CAD build for the part. Positions are in the model's coordinates, mm. Coordinates: 2 decimals unless noted, no trailing zeros. Write each loop counter-clockwise with the first axis right and the second up, starting at its lowest first coordinate (ties: lowest second). Pieces come first, ordered by that corner, then holes. Notation, with made-up numbers: (59.5, 61) -> (107.5, 61) arc R22 cw to (107.5, 92) -> close; hole circle Ø3 at (-24.5, 74.5). An arc over 180 degrees is marked (long way). Answer as CSV lines item,"result".
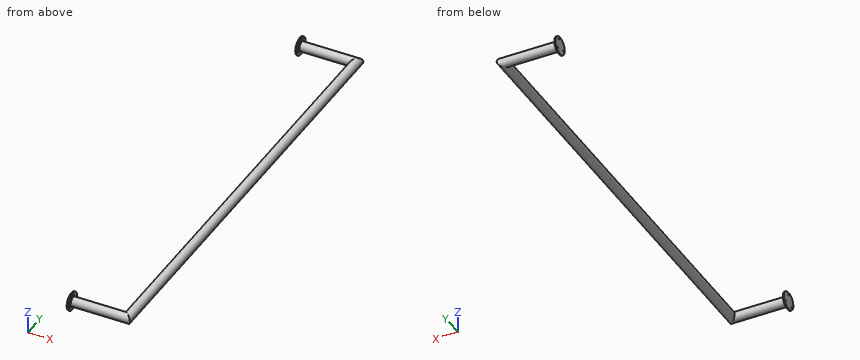
```python
from build123d import *

# Parameters (mm, degrees)
F0_R     = 21
F0_R_2   = 20
F3_R     = 40
F3_R_2   = 3.25
F4_DEPTH = 5
F5_SIZE  = 2
F6_SIZE  = 3


with BuildPart() as f2:
    # F2: sweep along a path in F1
    with BuildLine(Plane.XY) as f2_path:
        Line((0, 0), (250, 0))
        Line((250, 0), (250, -1948.319))
        Line((250, -1948.319), (0, -1948.319))
    # F0 (on Right) → F2 (sweep)
    with BuildSketch(Plane.YZ):
        Circle(F0_R)
        Circle(F0_R_2, mode=Mode.SUBTRACT)
    sweep(path=f2_path.line, transition=Transition.RIGHT)

    # F3 (on face) → F4 (join)
    with BuildSketch(Plane(origin=(0, 0, 0), x_dir=(0, -1, 0), z_dir=(-1, 0, 0))):
        with Locations((1948.319, 0)):
            Circle(F3_R)
        with Locations((1921.9052251846, -15.25)):
            Circle(F3_R_2, mode=Mode.SUBTRACT)
        with Locations((1974.7327748154, -15.25)):
            Circle(F3_R_2, mode=Mode.SUBTRACT)
        with Locations((1948.319, 30.5)):
            Circle(F3_R_2, mode=Mode.SUBTRACT)
        Circle(F3_R)
        with Locations((-21.187080299, -21.9398639103)):
            Circle(F3_R_2, mode=Mode.SUBTRACT)
        with Locations((29.5940196514, -7.3786178158)):
            Circle(F3_R_2, mode=Mode.SUBTRACT)
        with Locations((-8.4069393524, 29.3184817261)):
            Circle(F3_R_2, mode=Mode.SUBTRACT)
    extrude(amount=-F4_DEPTH)

    # F5
    f5_edges = [f2.edges().sort_by_distance(p)[0] for p in [
        (5, 11.656939, 29.318482),
        (5, -26.34402, -7.378618),
        (5, 24.43708, -21.939864),
        (5, -1945.069, 30.5),
        (5, -1971.482775, -15.25),
        (5, -1918.655225, -15.25),
    ]]
    chamfer(f5_edges, length=F5_SIZE)

    # F6
    f6_edges = [f2.edges().sort_by_distance(p)[0] for p in [
        (5, -21, 0),
        (5, -1927.319, 0),
    ]]
    chamfer(f6_edges, length=F6_SIZE)


solid = f2.part
```
Item 1: Saw through at B-B on y = -1611. Give the cut face in (x, z), and give its area (3 significant figures).
Answer below:
outline,"circle Ø42 at (250, 0); hole circle Ø40 at (250, 0)"
area,"129 mm2"
Item 2: Saw through at A-A on x = 158. Give the cut face in (y, z).
Answer below:
outline,"circle Ø42 at (-1948.32, 0); circle Ø42 at (0, 0); hole circle Ø40 at (-1948.32, 0); hole circle Ø40 at (0, 0)"
Item 3: Flat gauge pins, fed straight in: pin 1 (8 mm diameter, centred on y = -572.5, z = -19, fed in from -X); pin 2 (6 mm diameter, centred on y = -1428.5, z = 3, fed in from -X); pin 3 (1.5 mm diameter, centred on y = -1363, z = -3, fed in from -X). Where does each tip first touch, or does it go through?
Answer below:
pin 1,"stops at x = 235.3"
pin 2,"stops at x = 229"
pin 3,"stops at x = 229.12"
Item 4: Wall check: line 1 (Y direction, x = 201, z = 0.5); line 2 (Y direction, x = 55.5, z = -18.5); line 3 (X direction, y = -1112.5, z = 0.5). Give the ranges that are in metal, low to high. Write a range as from..to.
Answer below:
line 1,"y = -1969.31..-1968.31, -1928.33..-1927.32, -20.99..-19.99, 19.99..20.99"
line 2,"y = -1958.26..-1955.92, -1940.72..-1938.38, -9.94..-7.6, 7.6..9.94"
line 3,"x = 229.01..230.01, 269.99..270.99"
